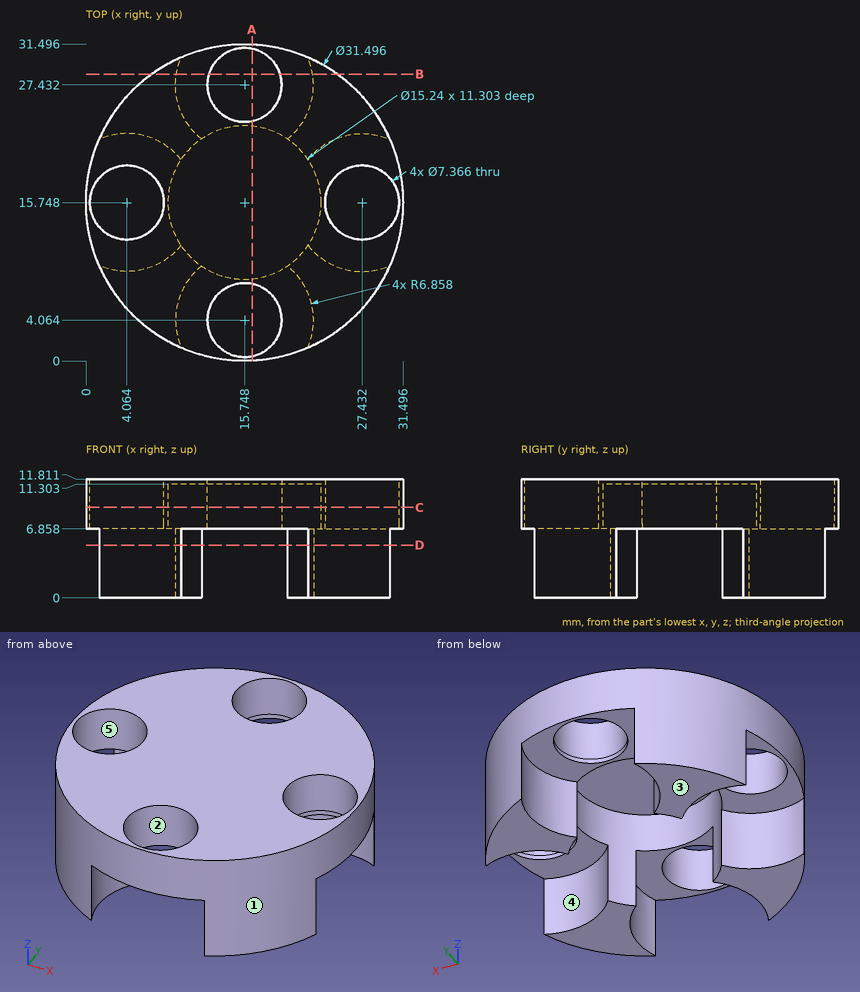
The figure shows three views and two pictorial views of one solid part (mm, origin at its lowest corner). Answer the questions. A direction names the side the tool comes from. Coordinates: 2 decimals unless noted, no trailing zeros. Loops run counter-clockwise (first coordinate to the right, second up) from the corner with the lowest first, then second, coordinate; pieces in that order, holes last. Notation, with made-up numbers: (50.25, -18.5) - (61.25, -18.5) arc R17 ccw to (61.25, 9.5) - close; hole circle Ø11 at (78, -8.75). An arc over 180 degrees is marked (long way). Use a Markdown table: item, result. Add a question column.
1) The part is cut by section C-C, the plane z = 9. Give the vertices of the cut face in (x, y) (3 decimals), and give its area (3 significant figures).
2) The part is cut by section A-A, the plane x = 16.5. Give the vertices of the cut face in (y, z), and give its area (3 significant figures).
3) The mould has two halves that part along Y. Classify the marked faces 1, 2 and 3: released by +Y, released by -Y, zero draft, split by the parting line, or undercut.
4) The part is cut by section D-D, the plane z = 5.25. Give the vertices of the cut face in (x, y).
5) Given pin 1 (12 mm diameter, centred on x = 15.748, y = 27.432, fed in from +Z); pin 2 (5 mm diameter, centred on y = 7, z = 1.5, fed in from +X); pin 3 (6 mm diameter, centred on x = 4.064, y = 15.748, fed in from -Z); pin 4 (3 mm diameter, centred on x = 27, y = 18.5, fed in from -Z), each flat-ended and moving along its own axis, determine where each tip first touches the part or whether it passes through.
6) The part is cut by section B-B, the plane y = 28.5. Give the vertices of the cut face in (x, z).
7) Find the intervals of material crossed by line 1 (Y direction, x = 18.5, z = 11.25); line 2 (X direction, y = 13.5, z = 10); line 3 (Y direction, x = 18, z = 11), in increasing order.
8) For the marked faces 4 and 5, determine the directions among +Z, -Z, +X, -X, +Y, -Y from which every point of the face is accessible in a straight line to the end or side of a thin tool.
Here are the results:
| question | item | result |
|---|---|---|
| 1 | outline | circle Ø31.496 at (15.748, 15.748); hole circle Ø7.366 at (4.064, 15.748); hole circle Ø15.24 at (15.748, 15.748); hole circle Ø7.366 at (15.748, 4.064); hole circle Ø7.366 at (15.748, 27.432); hole circle Ø7.366 at (27.432, 15.748) |
| 1 | area | 426 mm^2 |
| 2 | outline | (0.02, 6.86) - (0.46, 6.86) - (0.46, 11.81) - (0.02, 11.81) - close; (7.67, 6.86) - (8.17, 6.86) - (8.17, 11.3) - (23.33, 11.3) - (23.33, 6.86) - (23.83, 6.86) - (23.83, 11.81) - (7.67, 11.81) - close; (31.04, 6.86) - (31.48, 6.86) - (31.48, 11.81) - (31.04, 11.81) - close |
| 2 | area | 17.0 mm^2 |
| 3 | face 1 | split by the parting line |
| 3 | face 2 | undercut |
| 3 | face 3 | zero draft |
| 4 | outline | (1.31, 9.47) arc R15.75 ccw to (9.47, 1.31) arc R6.86 cw to (11.48, 9.43) arc R7.62 cw to (9.43, 11.48) arc R6.86 cw to start; (1.31, 22.03) arc R6.86 cw to (9.43, 20.01) arc R7.62 cw to (11.48, 22.06) arc R6.86 cw to (9.47, 30.19) arc R15.75 ccw to start; (20.01, 9.43) arc R6.86 cw to (22.03, 1.31) arc R15.75 ccw to (30.19, 9.47) arc R6.86 cw to (22.06, 11.48) arc R7.62 cw to start; (20.01, 22.06) arc R7.62 cw to (22.06, 20.01) arc R6.86 cw to (30.19, 22.03) arc R15.75 ccw to (22.03, 30.19) arc R6.86 cw to start |
| 5 | pin 1 | stops at z = 11.81 |
| 5 | pin 2 | stops at x = 30.19 |
| 5 | pin 3 | passes through |
| 5 | pin 4 | stops at z = 6.86 |
| 6 | outline | (6.51, 0) - (8.97, 0) - (8.97, 6.86) - (12.22, 6.86) - (12.22, 11.81) - (6.51, 11.81) - close; (19.27, 6.86) - (22.52, 6.86) - (22.52, 0) - (24.99, 0) - (24.99, 11.81) - (19.27, 11.81) - close |
| 7 | line 1 | y = 0.24 to 1.62, 6.51 to 8.64, 22.85 to 24.98, 29.88 to 31.25 |
| 7 | line 2 | x = 0.16 to 1.15, 6.98 to 8.47, 23.03 to 24.51, 30.35 to 31.33 |
| 7 | line 3 | y = 0.16 to 1.15, 6.98 to 8.47, 23.03 to 24.52, 30.35 to 31.33 |
| 8 | face 4 | -Z |
| 8 | face 5 | +Z, -Z |
